For this review, use the dimensioned drawing (mm, ordinates from the lowest corner) and the shaded views. A direction names the side the tool comes from. Coordinates: 2 decimals unless noted, no trailing zeros. Write each loop counter-clockwise with the first axis right and the second up, starting at its lowest first coordinate (ties: lowest second). Pieces come first, ordered by that corner, then holes. Notation, with made-up numbers: (22.5, 61.25) -> (33.5, 61.25) arc R30 cw to (33.5, 92.25) -> close; hole circle Ø11 at (83, 63). An arc over 180 degrees is marked (long way). Return JSON: item names as keys, results as strings. Group by question number.
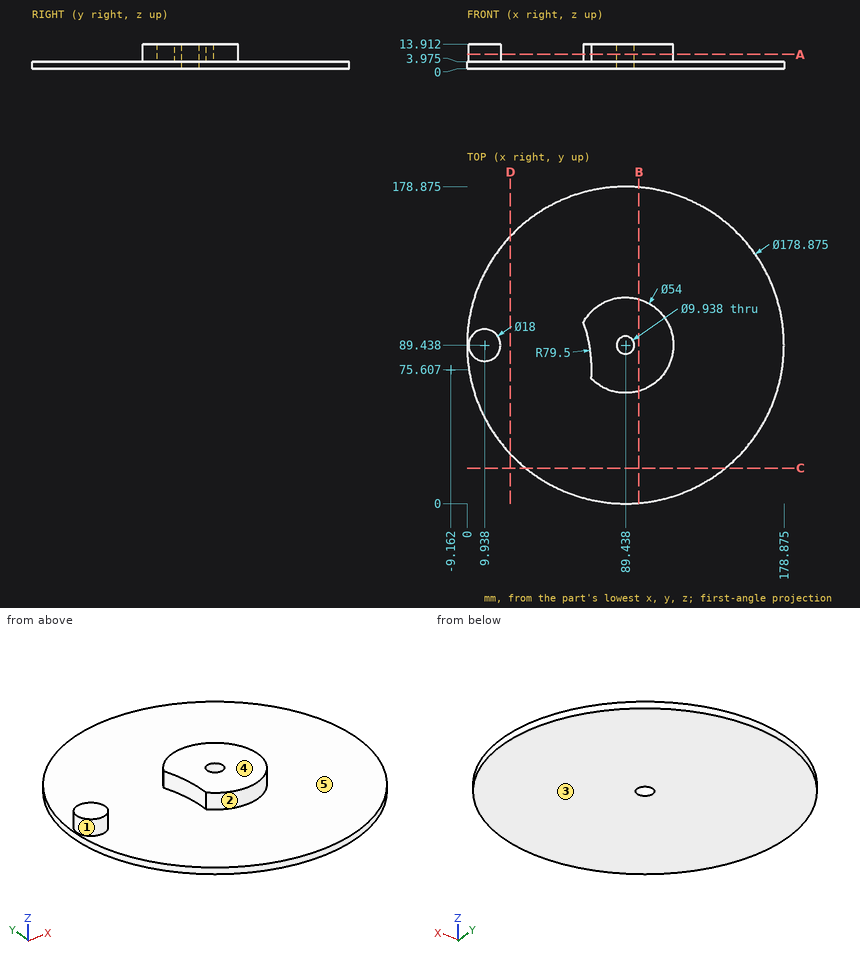
Q1. We need section A-A on z = 8. Write out the cut boundary in (x, y) (1 decimal).
Q2. The part is to be moulded in two halves that separate along X. For the marked faces 1, 2 and 3, say which applies: +X half, -X half, draft (parallel to the pull), parting line (faces both ways), or undercut.
Q3. We need section D-D on x = 24.5. Write out the cut boundary in (y, z) (1 decimal).
Q4. We need section B-B on x = 97. Write out the cut boundary in (y, z) (1 decimal).
Q5. For the marked faces 4 and 5, list the 3-axis set-ups (+Z, -Z, +X, -X, +Y, -Y) from which the entire face can be reached by the end or side of a thin tool; tool diameter is ignored.
Q6. For P1, Ø8, axis at y = 25, z = 3, coming from the -X side; P2, Ø2, axis at y = 88.5, z = 11, coming from the -X side; P3, Ø3, axis at x = 111, z = 2, coming from the +Y side (1 decimal), all flat-tipped, find the tip position at first contact; note any pin that passes through.
Q7. We need section C-C on y = 20. Write out the cut boundary in (x, z) (1 decimal).
Q8. Wall thickness on L1, parallel to Z at x = 151.5, y = 103.5 (1 decimal); L2, parallel to Y at x = 38.5, z = 2.25; L3, parallel to X at y = 23, z = 3.75 (1 decimal): over which ranges is each line inside the solid? List them lowest first.
Findings below:
{
 "1": {"outline": "circle Ø18 at (9.9, 89.4); (65.7, 102.3) arc R79.5 cw to (70.2, 70.5) arc R27 ccw (long way) to start; hole circle Ø9.9 at (89.4, 89.4)"},
 "2": {"face 1": "undercut", "face 2": "parting line", "face 3": "draft"},
 "3": {"outline": "(27.9, 0) -> (150.9, 0) -> (150.9, 4) -> (27.9, 4) -> close"},
 "4": {"outline": "(0.3, 0) -> (178.6, 0) -> (178.6, 4) -> (115.4, 4) -> (115.4, 13.9) -> (63.5, 13.9) -> (63.5, 4) -> (0.3, 4) -> close"},
 "5": {"face 4": "+Z, +X, -X, +Y, -Y", "face 5": "+Z"},
 "6": {"P1": "stops at x = 23.51", "P2": "stops at x = 0.94", "P3": "stops at y = 176.6"},
 "7": {"outline": "(33.1, 0) -> (145.8, 0) -> (145.8, 4) -> (33.1, 4) -> close"},
 "8": {"L1": "z = 0 to 4", "L2": "y = 15.92 to 162.95", "L3": "x = 29.6 to 149.3"}
}
